```python
from build123d import *

# Parameters (mm, degrees)
SKETCH1_R      = 1.5875
EXTRUDE1_DEPTH = 8.255
SKETCH2_R      = 2.413
EXTRUDE2_DEPTH = 0.635
SKETCH3_R      = 1.5875
EXTRUDE3_DEPTH = 5.08


with BuildPart() as part:
    # Sketch1 → Extrude1 (new body)
    with BuildSketch(Plane(origin=(0, 0, 0), x_dir=(1, 0, 0), z_dir=(0, 1, 0))):
        Circle(SKETCH1_R)
    extrude(amount=EXTRUDE1_DEPTH)

    # Sketch2 → Extrude2 (add, symmetric)
    with BuildSketch(Plane.XY):
        with BuildLine():
            Line((-3.81, 19.05), (-3.81, 7.62))
            Line((-3.81, 7.62), (3.81, 7.62))
            Line((3.81, 7.62), (3.81, 19.05))
            ThreePointArc((3.81, 19.05), (0, 22.86), (-3.81, 19.05))
        make_face()
        with Locations((0, 19.05)):
            Circle(SKETCH2_R, mode=Mode.SUBTRACT)
    extrude(amount=EXTRUDE2_DEPTH, both=True)

    # Sketch3 → Extrude3 (add)
    with BuildSketch(Plane.XZ):
        Circle(SKETCH3_R)
    extrude(amount=EXTRUDE3_DEPTH)


solid = part.part
```
Can you work these out from the model? Positions are in its coordinate system, mm. A direction names the side the tool comes from. Give positions to 0.01 mm unless a question says otherwise; leave off trailing zeros. Loops run counter-clockwise (first coordinate to the right, second up) from the corner with the lowest first, then second, coordinate; pieces in that order, holes last. Notation, with made-up numbers: M -28,-9.5 L 21,-9.5 A21 cw 21,28.5 Z; hole C 34.25,69 d10. An arc over 180 degrees is marked long. Use CSV: the item, a comma, the result in double quotes. Start each with the question number.
1. If I drill on L1, parallel to Y at x = 0, z = 0.15; L2, parallel to Z at x = -2.25, y = 9 (3 decimals); L3, parallel to Y at x = 1.5, z = 0, over which ranges is the centre line in solid material (lowest first)?
2. Imagine slicing it at D-D, the plane y = 1.5. Write out the boundary of the cut face in (x, z) (1 decimal).
3. For P1, Ø1.5, axis at x = 2, z = -0.5, coming from the -Y side; P2, Ø4, axis at x = 0, y = 19.05, coming from the +Z side; P3, Ø1.5, axis at y = 4, z = 0.5, coming from the -X side; P4, Ø1, axis at y = -1.5, z = 0, coming from the +X side, each with a flat end and sliding along its axis, tell me the tip position at first contact or that it passes through.
4. Imagine slicing it at C-C, the plane x = 2. Write out the boundary of the cut face in (y, z) (3 decimals).
5. On a 3-axis mill with a long thin cutter (end or side, diameter ignored), from which of +Z, -Z, +X, -X, +Y, -Y can I reach the whole of each face in a straight line? I mean faces 1 (the face through (3.81, 13, 0)), 2 (the face through (0, 8.255, 1)), 3 (the face through (0, 8.255, -1)), 4 (the face through (-0.34, 1.68, -1.55)). Say none if no direction works.
6. Imagine slicing it at B-B, the plane z = 0. Write out the boundary of the cut face in (x, y).
7. Imagine slicing it at A-A, the plane x = 0. Write out the boundary of the cut face in (y, z) (1 decimal).
8. If we mould it in two halves opening along Y, with no side actions, what happens to faces 5 (the face through (-0.314, 21.442, -0.009)), 6 (the face through (0.08, 22.86, 0.01)), 7 (the face through (3, 7.62, 0)), 8 (the face through (0, 14, -0.635))? For each: released by +Y, released by -Y, zero draft, split by the parting line, or undercut.
Response values:
1,L1,"-5.08 to 16.64, 21.46 to 22.86"
1,L2,"-0.635 to 0.635"
1,L3,"-5.08 to 17.16, 20.94 to 22.55"
2,outline,"C 0,0 d3.2"
3,P1,"y = -5.08"
3,P2,"through"
3,P3,"x = -1.59"
3,P4,"x = 1.59"
4,outline,"M 7.62,-0.635 L 17.7,-0.635 L 17.7,0.635 L 7.62,0.635 Z; M 20.4,-0.635 L 22.293,-0.635 L 22.293,0.635 L 20.4,0.635 Z"
5,face 1,"+Z, -Z, +X, +Y, -Y"
5,face 2,"+Z, +X, -X, +Y"
5,face 3,"-Z, +X, -X, +Y"
5,face 4,"-Y"
6,outline,"M -3.81,7.62 L -1.59,7.62 L -1.59,-5.08 L 1.59,-5.08 L 1.59,7.62 L 3.81,7.62 L 3.81,19.05 A3.81 ccw -3.81,19.05 Z; hole C 0,19.05 d4.83"
7,outline,"M -5.1,-1.6 L 8.3,-1.6 L 8.3,-0.6 L 16.6,-0.6 L 16.6,0.6 L 8.3,0.6 L 8.3,1.6 L -5.1,1.6 Z; M 21.5,-0.6 L 22.9,-0.6 L 22.9,0.6 L 21.5,0.6 Z"
8,face 5,"undercut"
8,face 6,"released by +Y"
8,face 7,"released by -Y"
8,face 8,"zero draft"
